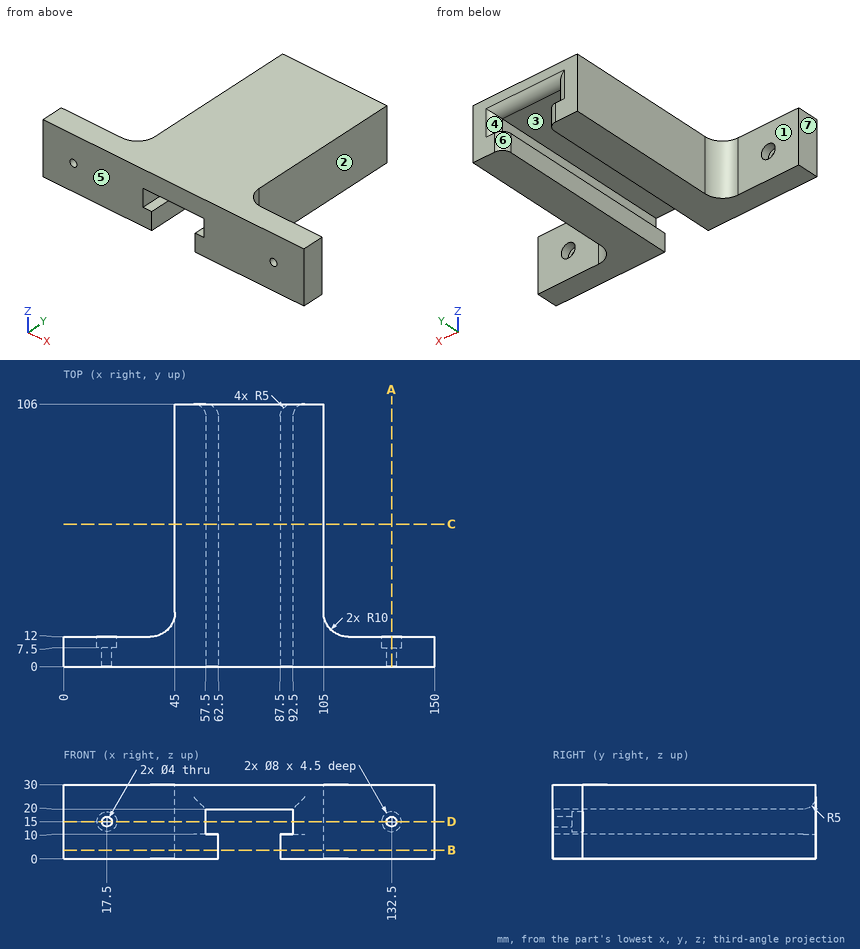
Verification items for this drawing (mm, ordinates from the low corner). A direction names the side the tool comes from. Coordinates: 2 decimals unless noted, no trailing zeros. Write each loop counter-clockwise with the first axis right and the second up, starting at its lowest first coordinate (ties: lowest second). Pieces come first, ordered by that corner, then holes. Notation, with made-up numbers: (68, 69.25) - (104, 69.25) arc R8 ccw to (104, 83.25) - close; hole circle Ø5 at (43, -7.5). An arc over 180 degrees is marked (long way). One line per question, with ' | ' between items.
Item 1: Sectioned sample at A-A on x = 132.5. Record the boundary of the cut face in (y, z).
Determined:
outline: (0, 0) - (12, 0) - (12, 11) - (7.5, 11) - (7.5, 13) - (0, 13) - close; (0, 17) - (7.5, 17) - (7.5, 19) - (12, 19) - (12, 30) - (0, 30) - close
Item 2: Gauge pin test, flat ends, axial feed: P1, Ø8, axis at y = 51.5, z = 2.5, coming from the -X side; P2, Ø6.5, axis at x = 19, z = 15, coming from the +Y side; P3, Ø8, axis at y = 54.5, z = 14.5, coming from the +X side. Record the tip position at first contact, or that the pin passes through.
Determined:
P1: stops at x = 45 | P2: stops at y = 12 | P3: stops at x = 105
Item 3: Sectioned sample at C-C on y = 57.5. Record the boundary of the cut face in (x, z).
Determined:
outline: (45, 0) - (62.5, 0) - (62.5, 10) - (57.5, 10) - (57.5, 20) - (92.5, 20) - (92.5, 10) - (87.5, 10) - (87.5, 0) - (105, 0) - (105, 30) - (45, 30) - close
Item 4: Sectioned sample at D-D on z = 15. Give the number of separate pieces and of enclosed holes in the cut face, plus the area to 3 significant figures.
Determined:
separate pieces: 4 | enclosed holes: 0 | area: 3,630 mm2
Item 5: Access from +Z, -Z, +X, -X, +Y, -Y to the whole of each face (thin tool, end or side, straight path). Record for the marked faces 1, 2, 3 and 4.
Determined:
face 1: +Z, -Z, -X, +Y | face 2: +Z, -Z, +X, +Y | face 3: +Y, -Y | face 4: +Y
Item 6: Thickness scan on line 1 (X direction, y = 9.95, z = 15); line 2 (X direction, y = 4, z = 15); line 3 (X direction, y = 31, z = 11). Record the ranges inside material, lowest first. Write a range as [from, to].
Determined:
line 1: x = [0, 13.5], [21.5, 57.5], [92.5, 128.5], [136.5, 150] | line 2: x = [0, 15.5], [19.5, 57.5], [92.5, 130.5], [134.5, 150] | line 3: x = [45, 57.5], [92.5, 105]
Item 7: Sectioned sample at B-B on z = 3.5. Record the boundary of the cut face in (x, y), plus the area to 3 significant figures.
Determined:
outline: (0, 0) - (62.5, 0) - (62.5, 101) arc R5 ccw to (57.5, 106) - (45, 106) - (45, 22) arc R10 cw to (35, 12) - (0, 12) - close; (87.5, 0) - (150, 0) - (150, 12) - (115, 12) arc R10 cw to (105, 22) - (105, 106) - (92.5, 106) arc R5 ccw to (87.5, 101) - close | area: 4,820 mm2
Item 8: Mould release check, pull along X, two halves, no side actions. Record for the marked faces 5, 6 and 7: pulls with the +X half, pulls with the -X half, needs draft (parallel to the pull), parting line crosses it, or undercut.
Determined:
face 5: needs draft | face 6: undercut | face 7: pulls with the -X half
